from build123d import *
from OCP.BRepAlgoAPI import BRepAlgoAPI_Cut
from OCP.TopTools import TopTools_ListOfShape

# Parameters (mm, degrees)
SKETCH1_R                 = 10
SKETCH1_R_2               = 1.35
BOSS_EXTRUDE1_DEPTH       = 3.175
SKETCH2_W                 = 38.058543228
SKETCH2_H                 = 41.75
SKETCH2_R                 = 1.35
BOSS_EXTRUDE2_DEPTH       = 3.175
SKETCH3_W                 = 38.058543228
SKETCH3_H                 = 41.75
SKETCH3_W_2               = 31.708543228
SKETCH3_H_2               = 35.4
BOSS_EXTRUDE3_DEPTH       = 20
FILLET1_R                 = 5
BOSS_EXTRUDE4_OUTLINE_R   = 1
BOSS_EXTRUDE4_OUTLINE_R_2 = 0.698520241
BOSS_EXTRUDE4_OUTLINE_R_3 = 0.699131638
BOSS_EXTRUDE4_DEPTH       = 4.524579022
SKETCH6_R                 = 0.699665004
SKETCH6_R_2               = 0.703272365
SKETCH6_R_3               = 0.700673295
SKETCH6_R_4               = 0.698053945
BOSS_EXTRUDE5_DEPTH       = 5.225420978
CUT_EXTRUDE3_DEPTH        = 39.629021569
CUT_EXTRUDE4_DEPTH        = 44.672508997


with BuildPart() as part:
    # Sketch1 → Boss-Extrude1 (new body)
    with BuildSketch(Plane(origin=(0, 0, 0), x_dir=(1, 0, 0), z_dir=(0, 1, 0))):
        with Locations(Location((0, 0, 0), (0, 0, 270))):
            Circle(SKETCH1_R)
        with Locations(Location((0, 7, 0), (0, 0, 270))):
            Circle(SKETCH1_R_2, mode=Mode.SUBTRACT)
        with Locations(Location((7, 0, 0), (0, 0, 270))):
            Circle(SKETCH1_R_2, mode=Mode.SUBTRACT)
        with Locations(Location((0, -7, 0), (0, 0, 270))):
            Circle(SKETCH1_R_2, mode=Mode.SUBTRACT)
        with Locations(Location((-7, 0, 0), (0, 0, 270))):
            Circle(SKETCH1_R_2, mode=Mode.SUBTRACT)
    extrude(amount=BOSS_EXTRUDE1_DEPTH)

    # Sketch2 → Boss-Extrude2 (add)
    with BuildSketch(Plane(origin=(0, 3.175, 0), x_dir=(1, 0, 0), z_dir=(0, 1, 0))):
        Rectangle(SKETCH2_W, SKETCH2_H)
        with Locations(Location((0, -7, 0), (0, 0, 270))):
            Circle(SKETCH2_R, mode=Mode.SUBTRACT)
        with Locations(Location((7, 0, 0), (0, 0, 270))):
            Circle(SKETCH2_R, mode=Mode.SUBTRACT)
        with Locations(Location((-7, 0, 0), (0, 0, 270))):
            Circle(SKETCH2_R, mode=Mode.SUBTRACT)
        with Locations(Location((0, 7, 0), (0, 0, 270))):
            Circle(SKETCH2_R, mode=Mode.SUBTRACT)
    extrude(amount=BOSS_EXTRUDE2_DEPTH)

    # Sketch3 → Boss-Extrude3 (add)
    with BuildSketch(Plane(origin=(0, 6.35, 0), x_dir=(1, 0, 0), z_dir=(0, 1, 0))):
        Rectangle(SKETCH3_W, SKETCH3_H)
        Rectangle(SKETCH3_W_2, SKETCH3_H_2, mode=Mode.SUBTRACT)
    extrude(amount=BOSS_EXTRUDE3_DEPTH)

    # Fillet1
    fillet1_edges = [part.edges().sort_by_distance(p)[0] for p in [
        (-19.029271614, 14.7625, -20.875),
        (-19.029271614, 14.7625, 20.875),
        (19.029271614, 14.7625, 20.875),
        (19.029271614, 14.7625, -20.875),
    ]]
    fillet(fillet1_edges, radius=FILLET1_R)

    # Boss-Extrude4: read off the stored shape, not the designer's step
    # Boss-Extrude4 outline → Boss-Extrude4 (add)
    # profile 1 of 2: a face of its own
    with BuildSketch(Plane.XY.offset(16.350420978)):
        with BuildLine():
            ThreePointArc((9.674791631, 35.998523082), (9.427181956, 35.932908065), (9.244559074, 35.753284112))
            ThreePointArc((9.244559074, 35.753284112), (8.147643376, 34.213929311), (6.807481387, 32.880961337))
            Line((6.807481387, 32.880961337), (6.807482447, 6.35))
            Line((6.807482447, 6.35), (11.963760646, 6.35))
            Line((11.963760646, 6.35), (11.963760646, 35.998520144))
            Line((11.963760646, 35.998520144), (9.674791631, 35.998523082))
        make_face()
        with Locations((9.857482447, 33.16)):
            Circle(BOSS_EXTRUDE4_OUTLINE_R, mode=Mode.SUBTRACT)
        with Locations((9.857482447, 12.46)):
            Circle(BOSS_EXTRUDE4_OUTLINE_R, mode=Mode.SUBTRACT)
    # profile 2 of 2: a face of its own
    with BuildSketch(Plane.XY.offset(16.350420978)):
        with BuildLine():
            Line((-12.751066043, 35.998520144), (-12.751066043, 6.35))
            Line((-12.751066043, 6.35), (-7.592517553, 6.35))
            Line((-7.592517553, 6.35), (-7.592516964, 32.880958857))
            ThreePointArc((-7.592516964, 32.880958857), (-8.932679762, 34.213927416), (-10.029597495, 35.753282149))
            ThreePointArc((-10.029597495, 35.753282149), (-10.212218516, 35.932905514), (-10.459826737, 35.998520144))
            Line((-10.459826737, 35.998520144), (-12.751066043, 35.998520144))
        make_face()
        with Locations((-10.642517553, 33.16)):
            Circle(BOSS_EXTRUDE4_OUTLINE_R_2, mode=Mode.SUBTRACT)
        with Locations((-10.642517553, 12.46)):
            Circle(BOSS_EXTRUDE4_OUTLINE_R_3, mode=Mode.SUBTRACT)
    extrude(amount=BOSS_EXTRUDE4_DEPTH)

    # Sketch6 → Boss-Extrude5 (add)
    with BuildSketch(Plane(origin=(0, 0, -15.649579022), x_dir=(-1, 0, 0), z_dir=(0, 0, -1))):
        with BuildLine():
            Line((10.992517553, 24.135), (10.992517553, 30.51))
            Line((10.992517553, 30.51), (7.192517366, 30.510000072))
            Line((7.192517366, 30.510000072), (6.892517553, 30.510000072))
            Line((6.892517553, 30.510000072), (6.892517553, 32.612557612))
            add(Edge.make_bspline(
                [(6.975743415, 32.783855976), (6.958921233, 32.771091761), (6.928542383, 32.73934935), (6.899316538, 32.679660552), (6.892517469, 32.634957243), (6.892517553, 32.612557612)],
                knots=[1.062e-06, 1.062e-06, 1.062e-06, 1.062e-06, 0.322323684, 0.658094096, 1, 1, 1, 1], degree=3, weights=[1, 1, 1, 1, 1, 1]))
            ThreePointArc((6.975743415, 32.783855976), (8.509170356, 34.198162413), (9.744817778, 35.878887355))
            add(Edge.make_bspline(
                [(9.950114528, 35.998516481), (9.923391157, 35.998516414), (9.869066225, 35.989019468), (9.796326784, 35.947026629), (9.759487209, 35.903468994), (9.744817778, 35.878887355)],
                knots=[0, 0, 0, 0, 0.324047023, 0.652881456, 1, 1, 1, 1], degree=3, weights=[1, 1, 1, 1, 1, 1]))
            Line((9.950114528, 35.998516481), (11.752517552, 35.998516481))
            Line((11.752517552, 35.998516481), (13.252517552, 35.998516481))
            Line((13.252517552, 35.998516481), (13.252517552, 6.318190736))
            Line((13.252517552, 6.318190736), (-12.46748245, 6.318190736))
            Line((-12.46748245, 6.318190736), (-12.46748245, 35.998516481))
            Line((-12.46748245, 35.998516481), (-10.96748245, 35.998516481))
            Line((-10.96748245, 35.998516481), (-9.165078771, 35.998516481))
            add(Edge.make_bspline(
                [(-8.959782959, 35.878887832), (-8.974454973, 35.903473814), (-9.011299786, 35.947034481), (-9.084041461, 35.989022268), (-9.138360889, 35.998516579), (-9.165078771, 35.998516481)],
                knots=[3.25e-07, 3.25e-07, 3.25e-07, 3.25e-07, 0.347182134, 0.676017862, 1, 1, 1, 1], degree=3, weights=[1, 1, 1, 1, 1, 1]))
            ThreePointArc((-8.959782959, 35.878887832), (-7.72413548, 34.198162669), (-6.190708414, 32.783856055))
            add(Edge.make_bspline(
                [(-6.107482447, 32.612555023), (-6.107481996, 32.634920643), (-6.114271613, 32.679614721), (-6.143476784, 32.739319032), (-6.173880837, 32.77108775), (-6.190708414, 32.783856055)],
                knots=[0, 0, 0, 0, 0.341381322, 0.677579946, 1, 1, 1, 1], degree=3, weights=[1, 1, 1, 1, 1, 1]))
            Line((-6.107482447, 32.612555023), (-6.107482447, 30.510000072))
            Line((-6.107482447, 30.510000072), (-6.407482262, 30.510000072))
            Line((-6.407482262, 30.510000072), (-10.207482447, 30.51))
            Line((-10.207482447, 30.51), (-10.207482447, 24.135))
            Line((-10.207482447, 24.135), (-9.049769141, 23.654765682))
            Line((-9.049769141, 23.654765682), (-9.049769141, 12.756914674))
            ThreePointArc((-9.049769141, 12.756914674), (-8.698297278, 11.908386539), (-7.849769141, 11.556914678))
            Line((-7.849769141, 11.556914678), (8.634804248, 11.556914678))
            ThreePointArc((8.634804248, 11.556914678), (9.483332385, 11.908386541), (9.834804247, 12.756914678))
            Line((9.834804247, 12.756914678), (9.834804247, 23.654765682))
            Line((9.834804247, 23.654765682), (10.992517553, 24.135))
        make_face()
        with Locations(Location((-9.857482447, 8.71, 0), (0, 0, 180))):
            Circle(SKETCH6_R, mode=Mode.SUBTRACT)
        with Locations(Location((-9.857482447, 33.16, 0), (0, 0, 180))):
            Circle(SKETCH6_R_2, mode=Mode.SUBTRACT)
        with Locations(Location((10.642517553, 33.16, 0), (0, 0, 180))):
            Circle(SKETCH6_R_3, mode=Mode.SUBTRACT)
        with Locations(Location((10.642517553, 8.71, 0), (0, 0, 180))):
            Circle(SKETCH6_R_4, mode=Mode.SUBTRACT)
    extrude(amount=BOSS_EXTRUDE5_DEPTH)

    # Sketch7 → Cut-Extrude3 (cut, through all)
    with BuildSketch(Plane(origin=(0, 26.35, 0), x_dir=(1, 0, 0), z_dir=(0, 1, 0))):
        Polygon((11.963760646, -16.350420978), (11.963760646, -22.528007323), (30.022930958, -23.761888284), (27.696884363, 28.84716935), (12.46748245, 20.875), (12.46748245, 15.649579022), (12.894365171, -16.350420978), align=None)
        Polygon((-12.751066043, -16.350420978), (-12.751066043, -23.761888284), (-21.517724294, -22.528007323), (-21.901635858, 22.206155736), (-13.252517552, 20.875), (-13.252517552, -16.350420978), align=None)
    extrude(amount=-CUT_EXTRUDE3_DEPTH, mode=Mode.SUBTRACT)


with BuildPart() as cut_extrude4_tool:
    # Sketch9 → Cut-Extrude4 (new, through all)
    with BuildSketch(Plane(origin=(-2e-09, 35.998516482, 0), x_dir=(1.0, 6.10309035182258e-11, 0), z_dir=(-6.10309035182258e-11, 1.0, -1.0368003232160358e-14))):
        Polygon((-12.751066041, -19.525420978), (13.891993445, -19.525420978), (13.555046053, -22.524424576), (-19.185008861, -22.524424576), align=None)
        Polygon((-13.25251755, 18.824579022), (15.127467216, 18.824579022), (13.105782864, 23.749676422), (-20.139693138, 23.131939537), align=None)
    extrude(amount=-CUT_EXTRUDE4_DEPTH)


with BuildPart() as part_1:
    add(part.part)

    # Cut-Extrude4: cut by cut_extrude4_tool, with a tolerance
    cut_extrude4_stock = TopTools_ListOfShape()
    cut_extrude4_stock.Append(part_1.part.wrapped)
    cut_extrude4_tools = TopTools_ListOfShape()
    cut_extrude4_tools.Append(cut_extrude4_tool.part.wrapped)
    cut_extrude4_cut = BRepAlgoAPI_Cut()
    cut_extrude4_cut.SetArguments(cut_extrude4_stock)
    cut_extrude4_cut.SetTools(cut_extrude4_tools)
    cut_extrude4_cut.SetFuzzyValue(0.00001)
    cut_extrude4_cut.Build()
    add(Compound.cast(cut_extrude4_cut.Shape()).solids(), mode=Mode.REPLACE)


solid = part_1.part
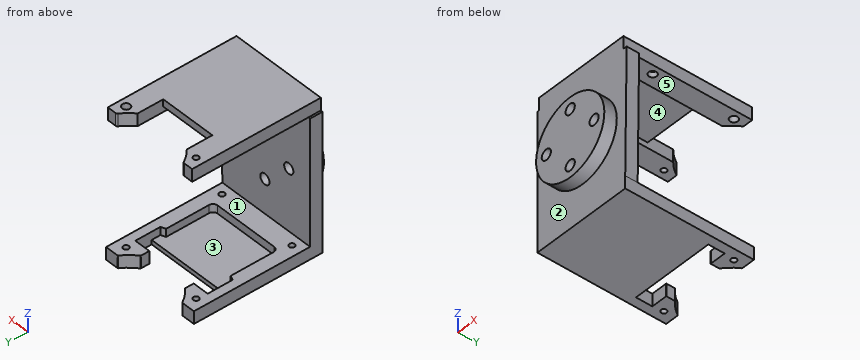
For this review, take the finished solid that the model builds, in its own axes (mm). Face numbers are marked on the shaded views. A direction names the side the tool comes from. Give positions to 0.01 mm unless a question says otherwise; leave off trailing zeros. Order: outer loops, then holes, each group sorted by start corner. A loop starts at its lowest first (then second) coordinate and runs counter-clockwise, first axis right, second up. Notation, with made-up numbers: (25, 70.25) - (38, 70.25) arc R27 cw to (38, 90.25) - close; hole circle Ø10 at (66, 0.25). An arc over 180 degrees is marked (long way). Answer as a JSON object with one key per item and string values. Group by question number.
Item 1: Take a section at A-A on y = 16.5. Give the boundary of the cut face in (x, z).
Item 2: Take a section at C-C on x = 0. Give the boundary of the cut face in (y, z) (3 decimals).
Item 3: Machinability: for the marked faces 1, 2 and 3, which of the approach directions +Z, -Z, +X, -X, +Y, -Y give a long, thin tool a straight path to every point of the face, cutting with its end or side? Answer none if there is none.
Item 4: Draft analysis for pull direction X (two halves, no side actions). For the marked faces 4 and 5, state which applies: pulls with the +X half, pulls with the -X half, needs draft (parallel to the pull), parting line crosses it, or undercut.
Item 5: Take a section at B-B on y = 30. Give the boundary of the cut face in (x, z), and give its area (3 significant figures).
Item 6: Take a section at D-D on z = -7. Give the boundary of the cut face in (x, y) (3 decimals), and give its area (3 significant figures).
Item 7: Clearance check with flat-ended pins moving along their axes: pin 1 Ø1 at (x, y) = (12.5, 4.5) entering from +Z; pin 2 Ø2.5 at (y, z) = (20, -16.5) entering from +X; pin 3 Ø5 at (y, z) = (29.5, 14) entering from +X. State where each tip first meets the part, or that it passes through.
Item 8: Wall thickness on line 1 along X through (y, z) = (8.71, -16.8); line 2 along X through (y, z) = (24.5, -16); line 3 along Z through (x, y) = (-9.75, 17.5): over which ranges is each line inside the solid? List them lowest first.
Reported:
{
 "1": {"outline": "(-13.25, -18.82) - (12.47, -18.82) - (12.47, -15.65) - (9.05, -15.65) - (9.05, -17.7) - (-9.83, -17.7) - (-9.83, -15.65) - (-13.25, -15.65) - close; (-12.75, 16.35) - (-7.59, 16.35) - (-7.59, 17.7) - (6.81, 17.7) - (6.81, 16.35) - (11.96, 16.35) - (11.96, 19.53) - (-12.75, 19.53) - close"},
 "2": {"outline": "(0, -10) - (3.175, -10) - (3.175, -18.825) - (26.35, -18.825) - (26.35, -17.7) - (11.557, -17.7) - (11.557, -15.65) - (6.35, -15.65) - (6.35, -8.35) - (0, -8.35) - close; (0, -5.65) - (6.35, -5.65) - (6.35, 5.65) - (0, 5.65) - close; (0, 8.35) - (6.35, 8.35) - (6.35, 17.7) - (26.35, 17.7) - (26.35, 19.525) - (3.175, 19.525) - (3.175, 10) - (0, 10) - close"},
 "3": {"face 1": "+X, -X, +Y", "face 2": "-Y", "face 3": "none"},
 "4": {"face 4": "undercut", "face 5": "needs draft"},
 "5": {"outline": "(-13.25, -18.82) - (-10.99, -18.82) - (-10.99, -15.65) - (-13.25, -15.65) - close; (-12.75, 16.35) - (-7.59, 16.35) - (-7.59, 19.53) - (-12.75, 19.53) - close; (6.81, 16.35) - (11.96, 16.35) - (11.96, 19.53) - (6.81, 19.53) - close; (10.21, -18.82) - (12.47, -18.82) - (12.47, -15.65) - (10.21, -15.65) - close", "area": "47.1 mm^2"},
 "6": {"outline": "(-13.253, 3.175) - (-7.141, 3.175) - (-7.141, 0) - (-1.35, 0) - (-1.35, 6.35) - (-13.253, 6.35) - close; (1.35, 0) - (7.141, 0) - (7.141, 3.175) - (12.583, 3.175) - (12.583, 6.35) - (1.35, 6.35) - close", "area": "110 mm^2"},
 "7": {"pin 1": "z = 16.35", "pin 2": "x = 12.47", "pin 3": "x = 11.96"},
 "8": {"line 1": "-13.25 to -11.34, -9.94 to 9.16, 10.56 to 12.47", "line 2": "-13.25 to -10.99, 10.21 to 12.47", "line 3": "-18.82 to -17.7, 16.35 to 19.53"}
}
